Autodesk Inventor part; units mm, degrees
ref_plane "YZ Plane" through (0, 0, 0) normal (1, 0, 0) x (0, 1, 0)
ref_plane "XZ Plane" through (0, 0, 0) normal (0, 1, 0) x (-1, 0, 0)
ref_plane "XY Plane" through (0, 0, 0) normal (0, 0, 1) x (1, 0, 0)
sketch "Sketch1" plane through (0, 0, 0) normal (0, 1, 0) x (-1, 0, 0)
  line L0 (0, 0) -> (0, -16.875) construction
  line L1 (0, -33.75) -> (16.875, -33.75) construction
  line L2 (33.75, -33.75) -> (33.75, -16.875) construction
  line L3 (33.75, 0) -> (16.875, 0) construction
  line L4 (33.75, -16.875) -> (0, -16.875) construction
  line L5 (16.875, -33.75) -> (16.875, 0) construction
  circle A0 centre (16.875, -16.875) radius 10.62
  line L6 (33.75, -16.875) -> (33.75, 0) construction
  line L7 (16.875, 0) -> (0, 0) construction
  line L8 (0, -16.875) -> (0, -33.75) construction
  line L9 (16.875, -33.75) -> (33.75, -33.75) construction
  line L10 (33.75, -25.3125) -> (25.3125, -33.75)
  line L11 (8.4375, -33.75) -> (0, -25.3125)
  line L12 (0, -8.4375) -> (8.4375, 0)
  line L13 (25.3125, 0) -> (33.75, -8.4375)
  line L14 (8.4375, 0) -> (25.3125, 0)
  line L15 (33.75, -8.4375) -> (33.75, -25.3125)
  line L16 (25.3125, -33.75) -> (8.4375, -33.75)
  line L17 (0, -25.3125) -> (0, -8.4375)
  dimension "d0" = 33.75
  dimension "d1" = 33.75
  dimension "d2" = 21.24
extrude "Extrusion1" add sketch "Sketch1" along normal blind 24.4
sketch "Sketch2" plane through (0, 0, 0) normal (0, -1, 0) x (1, 0, 0)
  circle A0 centre (-16.875, -16.875) radius 10.62
  point P0 (0, 0)
extrude "Extrusion2" add sketch "Sketch2" against normal blind 4
properties part number "dummy gopro nickle holder"
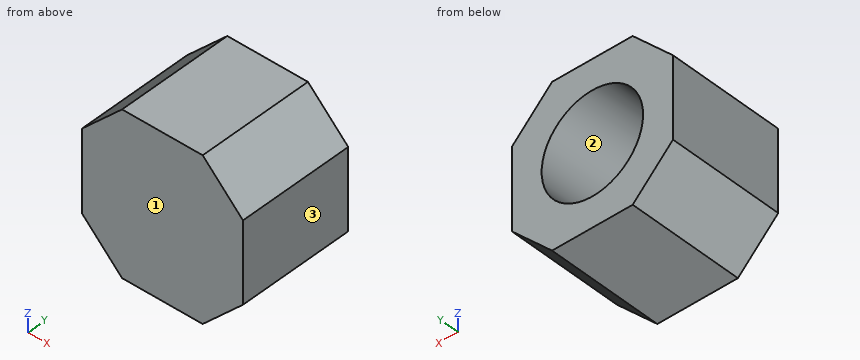
Model file for the job. Use its own axes, mm. Face numbers are marked on the shaded views. Round coordinates to 2 decimals unless told otherwise and drop trailing zeros. Loops run counter-clockwise (first coordinate to the right, second up) from the corner with the lowest first, then second, coordinate; pieces in that order, holes last. Notation, with made-up numbers: (-7, -3.5) -> (49, -3.5) arc R13 ccw to (49, 15.5) -> close; hole circle Ø7 at (64, -24). An arc over 180 degrees is marked (long way). Answer as CSV lines item,"result". Start each with the question number.
1) Probe line 1 along Z through (x, y) = (-12.5, 15.5); line 2 along Y through (x, z) = (-25.5, -14); line 3 along X through (y, z) = (7.5, -11). List the from-to ranges inside material, lowest first.
2) Slice it at C-C (x = -3). List the corners of the cut face in (y, z).
3) Slice it at A-A (z = -27). List the corners of the cut face in (x, y), plus the area to 3 significant figures.
4) Slice it at D-D (z = -20). List the corners of the cut face in (x, y).
5) Mould opens along X. For the marked faces 1, 2 and 3 say: +X half, -X half, draft (parallel to the pull), parting line (faces both ways), or undercut.
Filled in:
1,line 1,"z = -33.75 to -26.55, -7.2 to 0"
1,line 2,"y = 0 to 4"
1,line 3,"x = -33.75 to -25.72, -8.03 to 0"
2,outline,"(0, -28.31) -> (24.4, -28.31) -> (24.4, -5.44) -> (0, -5.44) -> close"
3,outline,"(-32.06, 0) -> (-1.69, 0) -> (-1.69, 24.4) -> (-13.67, 24.4) -> (-13.67, 4) -> (-20.08, 4) -> (-20.08, 24.4) -> (-32.06, 24.4) -> close"
3,area,"610 mm2"
4,outline,"(-33.75, 0) -> (0, 0) -> (0, 24.4) -> (-6.73, 24.4) -> (-6.73, 4) -> (-27.02, 4) -> (-27.02, 24.4) -> (-33.75, 24.4) -> close"
5,face 1,"draft"
5,face 2,"undercut"
5,face 3,"+X half"
